Source: CAD feature listing. Evaluate the final solid. Frame: model axes, mm. Round coordinates to 2 decimals unless told otherwise and drop trailing zeros. Loops run counter-clockwise (first coordinate to the right, second up) from the corner with the lowest first, then second, coordinate; pieces in that order, holes last. Notation, with made-up numbers: (2, 41.5) -> (59, 41.5) arc R18 ccw to (59, 48.5) -> close; hole circle Ø9 at (7, 11). An arc over 180 degrees is marked (long way). Put each result on its own line as item: value. Start each with the question number.
1. Cut plane D-D (x = 4). Return the cut outline in (y, z), then the cut area to 3 significant figures.
2. Contact query for flat-ended pins moving along their axis: pin 1 (3 mm diameter, centred on x = 6, y = 0, fed in from -Z); pin 2 (1 mm diameter, centred on x = -3.5, z = 3, fed in from -Y); pin 3 (1.5 mm diameter, centred on y = 0.5, z = 0.5, fed in from +X). Output: stop coordinate, or through.
3. Cut plane C-C (x = -6). Return the cut outline in (y, z).
4. Cut plane A-A (y = 0). Return the cut outline in (x, z), then the cut area to 3 significant figures.
5. Material intervals for L1, parallel to Z at x = 3.5, y = 0; L2, parallel to Z at x = 2.75, y = 0, sorted ascending.
```python
from build123d import *

# Parameters (mm, degrees)
SKETCH3_R          = 1.5
CUT_EXTRUDE1_DEPTH = 10


with BuildPart() as part:
    # Sketch2 → Revolve1 (revolve)
    with BuildSketch(Plane(origin=(0, 0, 0), x_dir=(1, 0, 0), z_dir=(0, 1, 0))):
        with BuildLine():
            Line((0, 0), (10, 0))
            ThreePointArc((10, 0), (7.071067812, 7.071067812), (0, 10))
            Line((0, 10), (0, 0))
        make_face()
    revolve1 = revolve(axis=Axis((0, 0, 0), (1, 0, 0)))

    # Mirror1: Revolve1 across plane
    add(revolve1.mirror(Plane(origin=(0, 0, 0), x_dir=(0, 0, 1), z_dir=(1, 0, 0))))

    # Sketch3 → Cut-Extrude1 (cut)
    with BuildSketch(Plane(origin=(0, 0, 0), x_dir=(0, 0, -1), z_dir=(1, 0, 0))):
        Circle(SKETCH3_R)
    extrude(amount=CUT_EXTRUDE1_DEPTH, mode=Mode.SUBTRACT)


solid = part.part
```
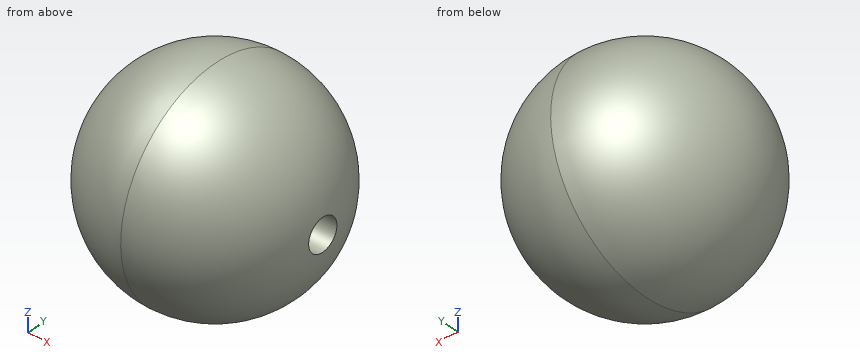
Solution:
1. outline: circle Ø18.33 at (0, 0); hole circle Ø3 at (0, 0)
1. area: 257 mm^2
2. pin 1: stops at z = -8.93
2. pin 2: stops at y = -9.12
2. pin 3: stops at x = 0
3. outline: circle Ø16 at (0, 0)
4. outline: (0, -1.5) -> (0, 1.5) -> (9.89, 1.5) arc R10 ccw (long way) to (9.89, -1.5) -> close
4. area: 284 mm^2
5. L1: z = -9.37 to -1.5, 1.5 to 9.37
5. L2: z = -9.61 to -1.5, 1.5 to 9.61
